Model file for the job. Use its own axes, mm. Face numbers are marked on the shaded views. A direction names the side the tool comes from. Give positions to 0.01 mm unless a question says otherwise; leave off trailing zeros. Loops run counter-clockwise (first coordinate to the right, second up) from the corner with the lowest first, then second, coordinate; pieces in that order, holes last. Notation, with made-up numbers: (21.25, 46) - (27.25, 46) arc R34 cw to (27.25, 80) - close; hole circle Ø6 at (12, 5). An arc over 180 degrees is marked (long way). Answer as CSV lines item,"result". Start each with the question number.
Item 1: Drill centre lines: L1, parallel to X at y = 2.25, z = 0.3; L2, parallel to Y at x = 8.75, z = 2; L3, parallel to Y at x = -5.75, z = 0.95. Where is each one in solid material? Low to high. Write a range as from..to.
Item 2: Tool access for the marked faces 1, 2 and 3: list every direction of +Z, -Z, +X, -X, +Y, -Y with a clear straight run to the whole face (end or side of a thin tool).
Item 3: Saw through at A-A on x = 0. Give the cut face in (y, z), plus the area to 3 significant figures.
Item 4: Pin check, flat tips, straight feed: pin 1 (3.5 mm diameter, centred on x = 0, y = 0, fed in from +Z); pin 2 (2 mm diameter, centred on x = 1.5, y = 2.5, fed in from -Z). Stop position of each tip, or through.
Item 5: Pull direction Y, two halves, no side cores. Call the marked faces 4, 5 and 6: pulls with the +Y half, pulls with the -Y half, needs draft (parallel to the pull), parting line crosses it, or undercut.
Item 6: Saw through at B-B on z = 0.9. State how many separate pieces and enclosed holes the cut face has, plus the area to 3 significant figures.
from build123d import *

# Parameters (mm, degrees)
MODEL_R             = 2.5
BOSS_EXTRUDE1_DEPTH = 4
SKETCH2_R           = 2.95
CUT_EXTRUDE1_DEPTH  = 4
SKETCH3_R           = 1.35
CUT_EXTRUDE2_DEPTH  = 4
CIRPATTERN1_COUNT   = 3


with BuildPart() as part:
    # Model → Boss-Extrude1 (new body)
    with BuildSketch(Plane.XY):
        with BuildLine():
            ThreePointArc((-11.997000624, 0.268283487), (-12, 0), (-11.997000624, -0.268283487))
            ThreePointArc((-11.997000624, -0.268283487), (-10.895606779, -0.741380557), (-9.707399683, -0.89966238))
            ThreePointArc((-9.707399683, -0.89966238), (-9.649769237, -1.387427358), (-9.56764597, -1.8716708))
            ThreePointArc((-9.56764597, -1.8716708), (-10.663129188, -2.358297721), (-11.586621996, -3.122529539))
            ThreePointArc((-11.586621996, -3.122529539), (-11.513915683, -3.380790682), (-11.43545361, -3.637361781))
            ThreePointArc((-11.43545361, -3.637361781), (-10.245387108, -3.780996591), (-9.060717605, -3.598110265))
            ThreePointArc((-9.060717605, -3.598110265), (-8.868002323, -4.049880962), (-8.652778483, -4.491372344))
            ThreePointArc((-8.652778483, -4.491372344), (-9.566788286, -5.266920743), (-10.237564162, -6.260373793))
            ThreePointArc((-10.237564162, -6.260373793), (-10.095042394, -6.487689809), (-9.947474154, -6.711762656))
            ThreePointArc((-9.947474154, -6.711762656), (-8.765147105, -6.514298768), (-7.679990073, -6.005060656))
            ThreePointArc((-7.679990073, -6.005060656), (-7.3678026, -6.384237295), (-7.036914342, -6.747209612))
            ThreePointArc((-7.036914342, -6.747209612), (-7.695403093, -7.74884917), (-8.059119765, -8.891039794))
            ThreePointArc((-8.059119765, -8.891039794), (-7.858328807, -9.068994892), (-7.653609502, -9.242416436))
            ThreePointArc((-7.653609502, -9.242416436), (-6.574807012, -8.719851201), (-5.67707542, -7.925516745))
            ThreePointArc((-5.67707542, -7.925516745), (-5.270707329, -8.201380692), (-4.850961252, -8.456428084))
            ThreePointArc((-4.850961252, -8.456428084), (-5.200582107, -9.603011921), (-5.227773414, -10.801406627))
            ThreePointArc((-5.227773414, -10.801406627), (-4.984980156, -10.915583944), (-4.739694926, -11.024304604))
            ThreePointArc((-4.739694926, -11.024304604), (-3.851815156, -10.218973149), (-3.214237879, -9.203894603))
            ThreePointArc((-3.214237879, -9.203894603), (-2.746610697, -9.354097), (-2.27201213, -9.480557045))
            ThreePointArc((-2.27201213, -9.480557045), (-2.284440889, -10.679195758), (-1.972903952, -11.836707735))
            ThreePointArc((-1.972903952, -11.836707735), (-1.707778059, -11.877857303), (-1.441798455, -11.913069177))
            ThreePointArc((-1.441798455, -11.913069177), (-0.816772145, -10.890214666), (-0.491001901, -9.736627657))
            ThreePointArc((-0.491001901, -9.736627657), (0, -9.749), (0.491001901, -9.736627657))
            ThreePointArc((0.491001901, -9.736627657), (0.816772145, -10.890214666), (1.441798455, -11.913069177))
            ThreePointArc((1.441798455, -11.913069177), (1.707778059, -11.877857303), (1.972903952, -11.836707735))
            ThreePointArc((1.972903952, -11.836707735), (2.284440889, -10.679195758), (2.27201213, -9.480557045))
            ThreePointArc((2.27201213, -9.480557045), (2.746610697, -9.354097), (3.214237879, -9.203894603))
            ThreePointArc((3.214237879, -9.203894603), (3.851815156, -10.218973149), (4.739694926, -11.024304604))
            ThreePointArc((4.739694926, -11.024304604), (4.984980156, -10.915583944), (5.227773414, -10.801406627))
            ThreePointArc((5.227773414, -10.801406627), (5.200582107, -9.603011921), (4.850961252, -8.456428084))
            ThreePointArc((4.850961252, -8.456428084), (5.270707329, -8.201380692), (5.67707542, -7.925516745))
            ThreePointArc((5.67707542, -7.925516745), (6.574807012, -8.719851201), (7.653609502, -9.242416436))
            ThreePointArc((7.653609502, -9.242416436), (7.858328807, -9.068994892), (8.059119765, -8.891039794))
            ThreePointArc((8.059119765, -8.891039794), (7.695403093, -7.74884917), (7.036914342, -6.747209612))
            ThreePointArc((7.036914342, -6.747209612), (7.3678026, -6.384237295), (7.679990073, -6.005060656))
            ThreePointArc((7.679990073, -6.005060656), (8.765147105, -6.514298768), (9.947474154, -6.711762656))
            ThreePointArc((9.947474154, -6.711762656), (10.095042394, -6.487689809), (10.237564162, -6.260373793))
            ThreePointArc((10.237564162, -6.260373793), (9.566788286, -5.266920743), (8.652778482, -4.491372344))
            ThreePointArc((8.652778482, -4.491372344), (8.868002323, -4.049880962), (9.060717605, -3.598110265))
            ThreePointArc((9.060717605, -3.598110265), (10.245387108, -3.780996591), (11.43545361, -3.637361781))
            ThreePointArc((11.43545361, -3.637361781), (11.513915683, -3.380790682), (11.586621996, -3.122529539))
            ThreePointArc((11.586621996, -3.122529539), (10.663129188, -2.358297721), (9.56764597, -1.8716708))
            ThreePointArc((9.56764597, -1.8716708), (9.649769237, -1.387427358), (9.707399683, -0.89966238))
            ThreePointArc((9.707399683, -0.89966238), (10.895606779, -0.741380557), (11.997000624, -0.268283487))
            ThreePointArc((11.997000624, -0.268283487), (12, 0), (11.997000624, 0.268283487))
            ThreePointArc((11.997000624, 0.268283487), (10.895606779, 0.741380557), (9.707399683, 0.89966238))
            ThreePointArc((9.707399683, 0.89966238), (9.649769237, 1.387427358), (9.56764597, 1.8716708))
            ThreePointArc((9.56764597, 1.8716708), (10.663129188, 2.358297721), (11.586621996, 3.122529539))
            ThreePointArc((11.586621996, 3.122529539), (11.513915683, 3.380790682), (11.43545361, 3.637361781))
            ThreePointArc((11.43545361, 3.637361781), (10.245387108, 3.780996591), (9.060717605, 3.598110265))
            ThreePointArc((9.060717605, 3.598110265), (8.868002323, 4.049880962), (8.652778483, 4.491372344))
            ThreePointArc((8.652778483, 4.491372344), (9.566788286, 5.266920743), (10.237564162, 6.260373793))
            ThreePointArc((10.237564162, 6.260373793), (10.095042394, 6.487689809), (9.947474154, 6.711762656))
            ThreePointArc((9.947474154, 6.711762656), (8.765147105, 6.514298768), (7.679990073, 6.005060656))
            ThreePointArc((7.679990073, 6.005060656), (7.3678026, 6.384237295), (7.036914342, 6.747209612))
            ThreePointArc((7.036914342, 6.747209612), (7.695403093, 7.74884917), (8.059119765, 8.891039794))
            ThreePointArc((8.059119765, 8.891039794), (7.858328807, 9.068994892), (7.653609502, 9.242416436))
            ThreePointArc((7.653609502, 9.242416436), (6.574807012, 8.719851201), (5.67707542, 7.925516745))
            ThreePointArc((5.67707542, 7.925516745), (5.270707329, 8.201380692), (4.850961252, 8.456428084))
            ThreePointArc((4.850961252, 8.456428084), (5.200582107, 9.603011921), (5.227773414, 10.801406627))
            ThreePointArc((5.227773414, 10.801406627), (4.984980156, 10.915583944), (4.739694926, 11.024304604))
            ThreePointArc((4.739694926, 11.024304604), (3.851815156, 10.218973149), (3.214237879, 9.203894603))
            ThreePointArc((3.214237879, 9.203894603), (2.746610697, 9.354097), (2.27201213, 9.480557045))
            ThreePointArc((2.27201213, 9.480557045), (2.284440889, 10.679195758), (1.972903952, 11.836707735))
            ThreePointArc((1.972903952, 11.836707735), (1.707778059, 11.877857303), (1.441798455, 11.913069177))
            ThreePointArc((1.441798455, 11.913069177), (0.816772145, 10.890214666), (0.491001901, 9.736627657))
            ThreePointArc((0.491001901, 9.736627657), (0, 9.749), (-0.491001901, 9.736627657))
            ThreePointArc((-0.491001901, 9.736627657), (-0.816772145, 10.890214666), (-1.441798455, 11.913069177))
            ThreePointArc((-1.441798455, 11.913069177), (-1.707778059, 11.877857303), (-1.972903952, 11.836707735))
            ThreePointArc((-1.972903952, 11.836707735), (-2.284440889, 10.679195758), (-2.27201213, 9.480557045))
            ThreePointArc((-2.27201213, 9.480557045), (-2.746610697, 9.354097), (-3.214237879, 9.203894603))
            ThreePointArc((-3.214237879, 9.203894603), (-3.851815156, 10.218973149), (-4.739694926, 11.024304604))
            ThreePointArc((-4.739694926, 11.024304604), (-4.984980156, 10.915583944), (-5.227773414, 10.801406627))
            ThreePointArc((-5.227773414, 10.801406627), (-5.200582107, 9.603011921), (-4.850961252, 8.456428084))
            ThreePointArc((-4.850961252, 8.456428084), (-5.270707329, 8.201380692), (-5.67707542, 7.925516745))
            ThreePointArc((-5.67707542, 7.925516745), (-6.574807012, 8.719851201), (-7.653609502, 9.242416436))
            ThreePointArc((-7.653609502, 9.242416436), (-7.858328807, 9.068994892), (-8.059119765, 8.891039794))
            ThreePointArc((-8.059119765, 8.891039794), (-7.695403093, 7.74884917), (-7.036914342, 6.747209612))
            ThreePointArc((-7.036914342, 6.747209612), (-7.3678026, 6.384237295), (-7.679990073, 6.005060656))
            ThreePointArc((-7.679990073, 6.005060656), (-8.765147105, 6.514298768), (-9.947474154, 6.711762656))
            ThreePointArc((-9.947474154, 6.711762656), (-10.095042394, 6.487689809), (-10.237564162, 6.260373793))
            ThreePointArc((-10.237564162, 6.260373793), (-9.566788286, 5.266920743), (-8.652778482, 4.491372344))
            ThreePointArc((-8.652778482, 4.491372344), (-8.868002323, 4.049880962), (-9.060717605, 3.598110265))
            ThreePointArc((-9.060717605, 3.598110265), (-10.245387108, 3.780996591), (-11.43545361, 3.637361781))
            ThreePointArc((-11.43545361, 3.637361781), (-11.513915683, 3.380790682), (-11.586621996, 3.122529539))
            ThreePointArc((-11.586621996, 3.122529539), (-10.663129188, 2.358297721), (-9.56764597, 1.8716708))
            ThreePointArc((-9.56764597, 1.8716708), (-9.649769237, 1.387427358), (-9.707399683, 0.89966238))
            ThreePointArc((-9.707399683, 0.89966238), (-10.895606779, 0.741380557), (-11.997000624, 0.268283487))
        make_face()
        Circle(MODEL_R, mode=Mode.SUBTRACT)
    extrude(amount=BOSS_EXTRUDE1_DEPTH)

    # Sketch2 → Cut-Extrude1 (cut)
    with BuildSketch(Plane.XY.offset(4)):
        Circle(SKETCH2_R)
    extrude(amount=-CUT_EXTRUDE1_DEPTH, mode=Mode.SUBTRACT)

    # Sketch3 → Cut-Extrude2 (cut)
    with BuildSketch(Plane.XY.offset(4)):
        with Locations((-5.638155725, 2.05212086)):
            Circle(SKETCH3_R)
    cut_extrude2 = extrude(amount=-CUT_EXTRUDE2_DEPTH, mode=Mode.SUBTRACT)

    # CirPattern1: Cut-Extrude2 ×3 about axis
    cirpattern1_axis = Axis((0, 0, 0), (0, 0, 1))
    for i in range(1, CIRPATTERN1_COUNT):
        add(cut_extrude2.rotate(cirpattern1_axis, i * 360 / CIRPATTERN1_COUNT), mode=Mode.SUBTRACT)


solid = part.part
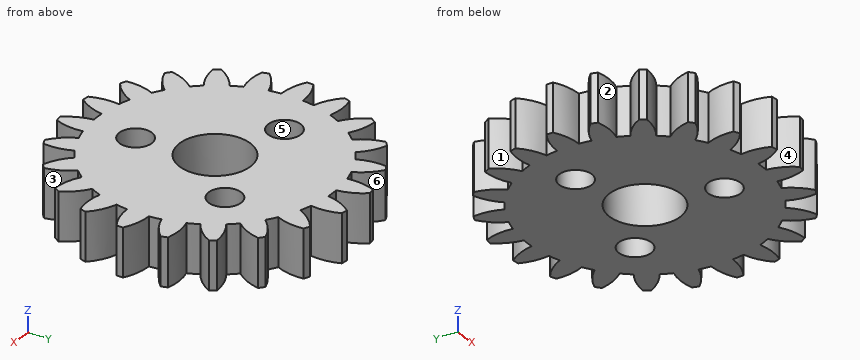
Responses:
1,L1,"-10.48..-6.97, -4.3..-1.91, 1.91..10.48"
1,L2,"-6.51..-4.56, -4.3..4.3, 4.56..6.51"
1,L3,"-8.01..0.71, 3.4..8.01"
2,face 1,"+Z, -Z, -X"
2,face 2,"+Z, -Z"
2,face 3,"+Z, -Z, +X"
3,outline,"(-9.75, 0) - (-6.77, 0) - (-6.77, 4) - (-9.75, 4) - close; (-5.05, 0) - (-2.95, 0) - (-2.95, 4) - (-5.05, 4) - close; (2.95, 0) - (9.75, 0) - (9.75, 4) - (2.95, 4) - close"
3,area,"47.5 mm2"
4,pin 1,"through"
4,pin 2,"z = 0"
5,face 4,"pulls with the -Y half"
5,face 5,"undercut"
5,face 6,"pulls with the +Y half"
6,separate pieces,"1"
6,enclosed holes,"4"
6,area,"323 mm2"
